Autodesk Inventor part; units mm, degrees
ref_plane "Work Plane1" through (2.6826, 0, 0) normal (0, 0.866, -0.5) x (-1, 0, 0)
ref_plane "YZ Plane" through (0, 0, 0) normal (1, 0, 0) x (0, 1, 0)
ref_plane "XZ Plane" through (0, 0, 0) normal (0, 1, 0) x (-1, 0, 0)
sketch "Boceto1" plane through (0, 0, 0) normal (1, 0, 0) x (0, 1, 0)
  line L0 (-2.0207, -3.5) -> (-4.0415, 0)
  line L1 (-4.0415, 0) -> (-2.0207, 3.5)
  line L2 (-2.0207, 3.5) -> (2.0207, 3.5)
  line L3 (2.0207, 3.5) -> (4.0415, 0)
  line L4 (4.0415, 0) -> (2.0207, -3.5)
  line L5 (2.0207, -3.5) -> (-2.0207, -3.5)
  point P0 (0, 0)
  point P1 (0, 0)
  dimension "d0" = 8.0829
extrude "Cuerpo" add sketch "Boceto1" along normal blind 3.2
sketch "Boceto2" plane through (0, 0, 0) normal (0, 0, 1) x (1, 0, 0)
  line L0 (3.2, 0) -> (8, 0)
  arc A0 (8, 0) -> (4.75, 3.25) centre (4.75, 0) ccw
  line L1 (4.75, 3.25) -> (3.2, 3.25)
  line L2 (3.2, -2.0207) -> (3.2, 2.0207)
  line L3 (3.2, 0) -> (3.2, 3.25)
  line L4 (2.1054, 0) -> (9.7677, 0)
  dimension "d8" = 3.25
  dimension "d9" = 4.8
revolve "Remate" add sketch "Boceto2" angle 360 about axis through (3.2, 0, 0) along (1, 0, 0)
sketch "Boceto3" plane through (0, 0, 0) normal (-1, 0, 0) x (0, 0, 1)
  line L0 (0, -5.658) -> (0, 5.658)
  line L1 (-4.9, 0) -> (4.9, 0)
  point P0 (0, 0)
hole "Rosca" at (0, 0, 0) direction (1, 0, 0) diameter 3.242 depth 5.3652 tip angle 120
sketch "Boceto4" plane through (0, 0, 0) normal (0, 0, 1) x (1, 0, 0)
  line L0 (0, 2.0207) -> (0, 4.0415)
  line L1 (0, 4.0415) -> (3.2, 4.0415)
  line L2 (3.2, 2.0207) -> (3.2, 4.0415)
  line L3 (-0.64, 0) -> (3.84, 0)
  line L4 (0.6302, 4.0415) -> (0, 2.95)
  line L5 (2.8874, 4.0415) -> (3.2, 3.5)
  dimension "d3" = 5.9
  dimension "d4" = 30
  dimension "d5" = 7
  dimension "d6" = 30
revolve "Chaflán1" cut sketch "Boceto4" angle 360 about axis through (-10, 0, 0) along (1, 0, 0)
chamfer "Chaflán2" distance 0.3789 angle 30 1 edges at (0, 0, -1.621) measured on face at (0, 2.4745, -0.3005)
ref_plane "Work Plane1" through (2.6826, 0, 0) normal (0, 0.866, -0.5) x (-1, 0, 0)
equation "\"d0\" = 1.1547 * SW"
equation "\"d1\" = SIH"
equation "\"d8\" = KR"
equation "\"d9\" = KOH1 - SIH"
equation "\"d11\" = GEL"
equation "\"d12\" = 1.02 * GEL"
equation "\"d3\" = SW0"
equation "\"d4\" = ANG1"
equation "\"d5\" = SW01"
equation "\"d6\" = ANG2"
equation "\"d14\" = -0.5 * GD1 + 0.5 * NND"
equation "\"d36\" = -0.5 * GD1 + 0.5 * NND"
equation "\"ANG1\" = 30deg"
equation "\"ANG2\" = 30deg"
equation "\"NND\" = 4"
equation "\"SIH\" = 3.2"
equation "\"KOH1\" = 8"
equation "\"GEL\" = 5.26"
equation "\"SW\" = 7"
equation "\"KR\" = 3.25"
equation "\"SW0\" = 5.9"
equation "\"SW01\" = SW"
equation "\"GUL\" = 0.541266 * PTC"
equation "\"THREADDIA\" = 4"
equation "\"TOA\" = 30deg"
equation "\"PTC\" = 0.7"
equation "\"E0\" = 1.155 * SW"
equation "\"GAL\" = 0.541266 * PTC"
properties part number "CF-TCA-0003" material "Acero, suave"
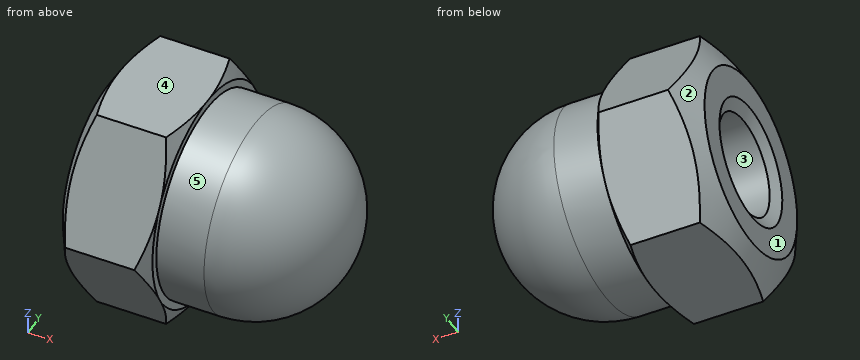
Could you check a few things on this model? Use its own coordinates, in mm. Face numbers are marked on the shaded views. A direction names the side the tool comes from. Coordinates: 2 decimals unless noted, no trailing zeros. Order: outer loops, then holes, each group sorted by start corner. A loop starts at its lowest first (then second) coordinate and runs counter-clockwise, first axis right, second up. Notation, with made-up numbers: (-8.5, 50.25) -> (43.5, 50.25) arc R5 ccw to (43.5, 55.25) -> close; hole circle Ø11 at (57.5, 33). An arc over 180 degrees is marked (long way). One line per item, written item: value. Start each with the question number.
1) Imagine slicing it at A-A on x = 3.5. List the corners of the cut face in (y, z) for me.
2) Imagine slicing it at B-B on x = 7.25. List the corners of the cut face in (y, z) for me.
3) If I drill on L1, parallel to Z at x = 1.5, y = 0; L2, parallel to Z at x = 3.6, y = 0; L3, parallel to Y at x = 4.25, z = -0.5, over which ranges is the centre line in solid material (lowest first)? Write a range as [from, to].
4) I'm going to push flat-ended pins straight in: pin 1 (2 mm diameter, centred on x = 5, y = -1, fed in from -Z); pin 2 (1.5 mm diameter, centred on x = 7, y = -1, fed in from +Z); pin 3 (3 mm diameter, centred on x = 5, z = 1, fed in from -Y). Where does each tip first touch, or does it pass through?
5) Which directions (+Z, -Z, +X, -X, +Y, -Y) give clear straight access to the entire face, cutting with the end or side of a thin tool? Please do the marked faces 4 and 5.
6) We'd pull the mould along Y, two halves only. Please class the marked faces 1, 2 and 3: +Y half, -Y half, draft (parallel to the pull), parting line (faces both ways), or undercut.
Answer list:
1. outline: circle Ø6.5 at (0, 0); hole circle Ø3.24 at (0, 0)
2. outline: circle Ø4.15 at (0, 0)
3. L1: z = [-3.5, -1.62], [1.62, 3.5]
3. L2: z = [-3.25, -1.62], [1.62, 3.25]
3. L3: y = [-3.21, -1.54], [1.54, 3.21]
4. pin 1: stops at z = -3.25
4. pin 2: stops at z = 2.76
4. pin 3: stops at y = -3.25
5. face 4: +Z, +X, -X, +Y, -Y
5. face 5: +X
6. face 1: draft
6. face 2: parting line
6. face 3: undercut
